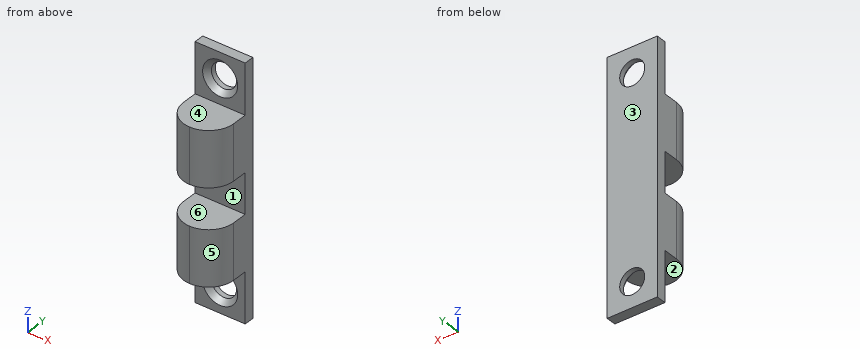
Autodesk Fusion 360 part; units mm, degrees
sketch "Sketch1" plane through (0, 0, 0) normal (0, 1, 0) x (1, 0, 0)
  line L0 (0, 0) -> (10, 0)
  line L1 (10, 0) -> (10, -50)
  line L2 (10, -50) -> (0, -50)
  line L3 (0, -50) -> (0, 0)
  dimension "d1" = 10
  dimension "d2" = 50
extrude "Extrude1" add sketch "Sketch1" against normal blind 2
sketch "Sketch2" plane through (0, -2, 0) normal (0, -1, 0) x (1, 0, 0)
  line L0 (10, 50) -> (0, 50)
  line L1 (0, 50) -> (0, 0)
  line L2 (0, 0) -> (10, 0)
  line L3 (10, 0) -> (10, 50)
  line L4 (0, 40) -> (10, 40)
  line L5 (10, 40) -> (10, 29)
  line L6 (10, 29) -> (0, 29)
  line L7 (0, 29) -> (0, 40)
  line L8 (0, 10) -> (10, 10)
  line L9 (10, 10) -> (10, 21)
  line L10 (10, 21) -> (0, 21)
  line L11 (0, 21) -> (0, 10)
  circle A0 centre (5, 45) radius 2.5
  circle A1 centre (5, 5) radius 2.5
  dimension "d5" = 5
  dimension "d6" = 5
  dimension "d7" = 5
  dimension "d8" = 5
  dimension "d9" = 11
  dimension "d10" = 11
  dimension "d11" = 10
  dimension "d12" = 10
  dimension "d13" = 8
  dimension "d14" = 5
  dimension "d15" = 5
  dimension "d16" = 5
extrude "Extrude2" add sketch "Sketch2" along normal blind 8 contours L1 L3 L4 L5 L6 L7 | L1 L3 L8 L9 L10 L11
extrude "Extrude3" cut sketch "Sketch2" against normal blind 2 contours A0 | A1
chamfer "Chamfer1" distance 1 angle 45 2 edges at (2.6692, -2, 45.904) (2.6692, -2, 5.904)
fillet "Fillet1" radius 5 4 edges at (0, -10, 34.5) (0, -10, 15.5) (10, -10, 34.5) (10, -10, 15.5)
Geometry check sheet. Reference: the model listing, model coordinates, mm. Face numbers are marked on the shaded views. A direction names the side the tool comes from. Round coordinates to 2 decimals unless told otherwise and drop trailing zeros. Loops run counter-clockwise (first coordinate to the right, second up) from the corner with the lowest first, then second, coordinate; pieces in that order, holes last. Notation, with made-up numbers: (70, 33) - (83, 33) arc R22 cw to (83, 60) - close; hole circle Ø9 at (52, 55). An arc over 180 degrees is marked (long way). Write item = value, one per line. Start each with the question number.
1. Depth check by flat-ended pin: pin 1 (2.5 mm diameter, centred on x = 3, y = -7, fed in from +Z); pin 2 (5 mm diameter, centred on x = 4.5, z = 44, fed in from -Y); pin 3 (1.5 mm diameter, centred on x = 7.5, z = 20.5, fed in from -Y). Enter the tip coordinate at first touch or a pass-through.
2. Section check B-B on y = -2.5. Enter the section's corners in (x, z), then the cut area to 3 significant figures.
3. Thickness scan on line 1 (Z direction, x = 5, y = -0.2); line 2 (Z direction, x = 2, y = -5.5); line 3 (Z direction, x = 4, y = -1.75). Record the ranges inside material, lowest first.
4. Section check D-D on y = -6. Enter the section's corners in (x, z), then the cut area to 3 significant figures.
5. Mould release check, pull along Z, two halves, no side actions. Record for the marked faces 4, 5 and 6: released by +Z, released by -Z, zero draft, split by the parting line, or undercut.
6. Section check A-A on z = 45. Enter the section's corners in (x, y).
7. Set-up check for the marked faces 1, 2 and 3: record each of +Z, -Z, +X, -X, +Y, -Y from which the full face is reachable in a straight line by a thin tool's end or side.
Working result:
q1.pin_1 = 40
q1.pin_2 = -2
q1.pin_3 = -9.68
q2.outline = (0, 10) - (10, 10) - (10, 21) - (0, 21) - close; (0, 29) - (10, 29) - (10, 40) - (0, 40) - close
q2.area = 220 mm^2
q3.line_1 = 0 to 2.5, 7.5 to 42.5, 47.5 to 50
q3.line_2 = 10 to 21, 29 to 40
q3.line_3 = 0 to 1.91, 8.09 to 41.91, 48.09 to 50
q4.outline = (0.1, 10) - (9.9, 10) - (9.9, 21) - (0.1, 21) - close; (0.1, 29) - (9.9, 29) - (9.9, 40) - (0.1, 40) - close
q4.area = 216 mm^2
q5.face_4 = released by +Z
q5.face_5 = zero draft
q5.face_6 = undercut
q6.outline = (0, -2) - (1.5, -2) - (2.5, -1) - (2.5, 0) - (0, 0) - close; (7.5, -1) - (8.5, -2) - (10, -2) - (10, 0) - (7.5, 0) - close
q7.face_1 = +X, -X, -Y
q7.face_2 = -Z, +X, -X, -Y
q7.face_3 = +Z, -Z, +X, -X, +Y
